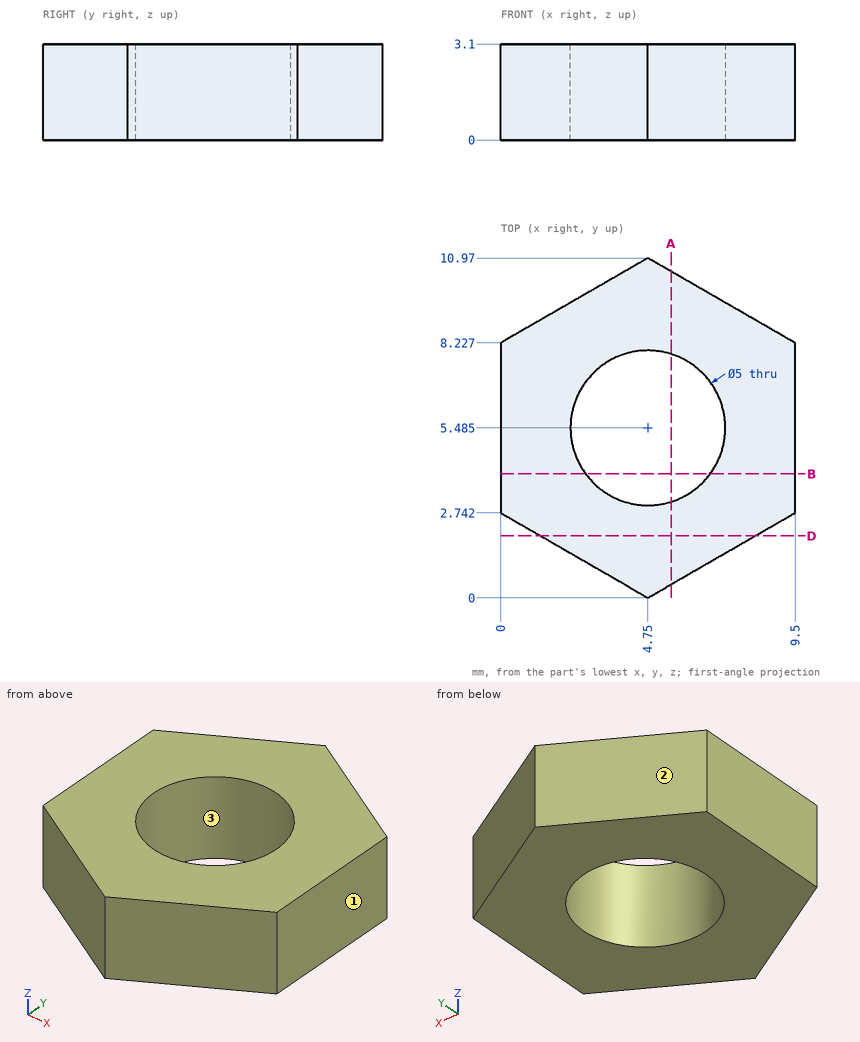
Geometry check sheet. Reference: drawing and pictorial views, mm from the part's lowest x, y, z. Give positions to 0.01 mm unless a question says otherwise; leave off trailing zeros. Loops run counter-clockwise (first coordinate to the right, second up) from the corner with the lowest first, then second, coordinate; pieces in that order, holes last. Notation, with made-up numbers: (24, -23.5) -> (46, -23.5) arc R19 cw to (46, 13.5) -> close; hole circle Ø1 at (37, -6.75). An arc over 180 degrees is marked (long way). Answer in a Markdown table with one row per item. Add a question column.
1) Gauge pin test, flat end, axial feed: P1, Ø4, axis at x = 4.75, y = 5.48, coming from the +Z side. Record the tip position at first contact, or that the pin passes through.
2) Cross-section at B-B on y = 4. Record the boundary of the cut face in (x, z), and give its area (3 significant figures).
3) Cross-section at D-D on y = 2. Record the boundary of the cut face in (x, z), and give its area (3 significant figures).
4) Material ranges on probe 1 along X at (y, z) = (4, 0.75); probe 2 along Y at (x, z) = (2.75, 2.2) (1 decimal); probe 3 along Y at (x, z) = (6.5, 1.5), recorded low to high. Write a range as from..to.
5) Draft check along X on the marked faces 1, 2 and 3. Enter one of: pulls with the +X half, pulls with the -X half, needs draft (parallel to the pull), parting line crosses it, or undercut.
6) Cross-section at A-A on x = 5.5. Record the boundary of the cut face in (y, z).
Outcome:
| question | item | result |
|---|---|---|
| 1 | P1 | passes through |
| 2 | outline | (0, 0) -> (2.74, 0) -> (2.74, 3.1) -> (0, 3.1) -> close; (6.76, 0) -> (9.5, 0) -> (9.5, 3.1) -> (6.76, 3.1) -> close |
| 2 | area | 17.0 mm^2 |
| 3 | outline | (1.29, 0) -> (8.21, 0) -> (8.21, 3.1) -> (1.29, 3.1) -> close |
| 3 | area | 21.5 mm^2 |
| 4 | probe 1 | x = 0..2.74, 6.76..9.5 |
| 4 | probe 2 | y = 1.2..4, 7..9.8 |
| 4 | probe 3 | y = 1.01..3.7, 7.27..9.96 |
| 5 | face 1 | pulls with the +X half |
| 5 | face 2 | pulls with the -X half |
| 5 | face 3 | undercut |
| 6 | outline | (0.43, 0) -> (3.1, 0) -> (3.1, 3.1) -> (0.43, 3.1) -> close; (7.87, 0) -> (10.54, 0) -> (10.54, 3.1) -> (7.87, 3.1) -> close |
